Source: CAD feature listing. Evaluate the final solid. Frame: model axes, mm. A direction names the side the tool comes from. Give positions to 0.01 mm unless a question says otherwise; leave off trailing zeros. Loops run counter-clockwise (first coordinate to the right, second up) from the corner with the lowest first, then second, coordinate; pieces in that order, holes last. Notation, with made-up numbers: M 42,-27 L 76,-27 A22 cw 76,-14 Z; hole C -19,-15.5 d3. An arc over 180 degrees is marked long. Answer in a Markdown table with one row per item.
```python
from build123d import *

# Parameters (mm, degrees)
F3_DEPTH = 7
F4_DEPTH = 1.6


with BuildPart() as f3:
    # F2 (on Front) → F3 (new body)
    with BuildSketch(Plane.XZ):
        with BuildLine():
            ThreePointArc((28.8, 75), (0, 103.8), (-28.8, 75))
            Line((-28.8, 75), (-28.8, 0))
            ThreePointArc((-28.8, 0), (0, -28.8), (28.8, 0))
            Line((28.8, 0), (28.8, 75))
        make_face()
        with BuildLine():
            Line((27.2, 75), (27.2, 0))
            ThreePointArc((27.2, 0), (0, -27.2), (-27.2, 0))
            Line((-27.2, 0), (-27.2, 75))
            ThreePointArc((-27.2, 75), (0, 102.2), (27.2, 75))
        make_face(mode=Mode.SUBTRACT)
    extrude(amount=F3_DEPTH)

    # F2 (on Front) → F4 (join)
    with BuildSketch(Plane.XZ):
        with BuildLine():
            ThreePointArc((28.8, 75), (0, 103.8), (-28.8, 75))
            Line((-28.8, 75), (-28.8, 0))
            ThreePointArc((-28.8, 0), (0, -28.8), (28.8, 0))
            Line((28.8, 0), (28.8, 75))
        make_face()
        with BuildLine():
            Line((27.2, 75), (27.2, 0))
            ThreePointArc((27.2, 0), (0, -27.2), (-27.2, 0))
            Line((-27.2, 0), (-27.2, 75))
            ThreePointArc((-27.2, 75), (0, 102.2), (27.2, 75))
        make_face(mode=Mode.SUBTRACT)
        with BuildLine():
            ThreePointArc((-27.2, 0), (0, -27.2), (27.2, 0))
            Line((27.2, 0), (27.2, 75))
            ThreePointArc((27.2, 75), (0, 102.2), (-27.2, 75))
            Line((-27.2, 75), (-27.2, 0))
        make_face()
    extrude(amount=-F4_DEPTH)


solid = f3.part
```
Q1. Contact query for flat-ended pins moving along their axis: pin 1 Ø1 at (x, z) = (0.5, 39.5) entering from -Y; pin 2 Ø4 at (x, y) = (3.5, 0.5) entering from +Z; pin 3 Ø1 at (x, y) = (19.5, 0) entering from +Z. Output: stop coordinate, or through.
Values follow:
| item | result |
|---|---|
| pin 1 | y = 0 |
| pin 2 | z = 103.76 |
| pin 3 | z = 96.64 |
Q2. Section query C-C (z = -17.5). Output: boundary loops of the cut face in (x, y), plus the area to 3 significant figures.
Values follow:
| item | result |
|---|---|
| outline | M -22.87,-7 L -20.82,-7 L -20.82,0 L 20.82,0 L 20.82,-7 L 22.87,-7 L 22.87,1.6 L -22.87,1.6 Z |
| area | 102 mm^2 |
Q3. Section query B-B (x = 0). Output: boundary loops of the cut face in (y, z).
Values follow:
| item | result |
|---|---|
| outline | M -7,-28.8 L 1.6,-28.8 L 1.6,103.8 L -7,103.8 L -7,102.2 L 0,102.2 L 0,-27.2 L -7,-27.2 Z |
Q4. Ray query, probe 1 along X at (y, z) = (-3.5, 30.5); probe 2 along Z at (x, y) = (0.5, -4.5); probe 3 along Y at (x, z) = (13.5, -9.5). Return the intervals inside material, ascending. Write a range as from..to.
Values follow:
| item | result |
|---|---|
| probe 1 | -28.8..-27.2, 27.2..28.8 |
| probe 2 | -28.8..-27.2, 102.2..103.8 |
| probe 3 | 0..1.6 |
Q5. Reachability of faces 4 (the flat face through (-27.2, -3, 37)), 5 (the flat face through (0, 1.6, 38)) from +Z, -Z, +X, -X, +Y, -Y: full face, straight path, thin tool, end or side. Return the list, or none.
Values follow:
| item | result |
|---|---|
| face 4 | -Y |
| face 5 | +Z, -Z, +X, -X, +Y |
Q6. Mould query, pull axis X, two halves, no side actions, for faces 1 (the flat face through (28.8, -3, 37)), 2 (the cylindrical face through (0.633, -2.76, 103.793)), 3 (the flat face through (27.2, -3, 38)). Classes: +X half, -X half, draft (parallel to the pull), parting line (faces both ways), or undercut.
Values follow:
| item | result |
|---|---|
| face 1 | +X half |
| face 2 | parting line |
| face 3 | undercut |
Q7. Section query A-A (y = -3.75). Output: boundary loops of the cut face in (x, z), plus the area to 3 significant figures.
Values follow:
| item | result |
|---|---|
| outline | M -28.8,0 A28.8 ccw 28.8,0 L 28.8,75 A28.8 ccw -28.8,75 Z; hole M -27.2,0 A27.2 ccw 27.2,0 L 27.2,75 A27.2 ccw -27.2,75 Z |
| area | 521 mm^2 |
